from build123d import *

# Parameters (mm, degrees)
F0_R           = 12.5
F1_DEPTH       = 122.5
F2_R           = 12.5
F3_DEPTH       = 65
F4_DEPTH       = 25
F5_DEPTH       = 25
F6_R           = 5.5
F7_DEPTH       = 30
F9_D           = 5.5
F9_DEPTH       = 100
F9_CSINK_D     = 11
F9_CSINK_ANGLE = 90


with BuildPart() as f1:
    # F0 (on Top) → F1 (new body)
    with BuildSketch(Plane.XY):
        Circle(F0_R)
    extrude(amount=F1_DEPTH)

    # F2 (on Right) → F3 (join)
    with BuildSketch(Plane.YZ):
        Circle(F2_R)
    extrude(amount=F3_DEPTH)

    # F2 (on Right) → F4 (join)
    with BuildSketch(Plane.YZ):
        Circle(F2_R)
    extrude(amount=-F4_DEPTH)

    # F0 (on Top) → F5 (join)
    with BuildSketch(Plane.XY):
        Circle(F0_R)
    extrude(amount=-F5_DEPTH)

    # F6 (on face) → F7 (cut)
    with BuildSketch(Plane(origin=(-25, 0, 0), x_dir=(0, -1, 0), z_dir=(-1, 0, 0))):
        Circle(F6_R)
    extrude(amount=-F7_DEPTH, mode=Mode.SUBTRACT)

    # F9
    with Locations(Plane(origin=(5, 0, 0), x_dir=(0, -1, 0), z_dir=(-1, 0, 0))):
        with Locations((0, 0)):
            CounterSinkHole(F9_D / 2, F9_CSINK_D / 2, depth=F9_DEPTH, counter_sink_angle=F9_CSINK_ANGLE)


solid = f1.part
Model file for the job. Use its own axes, mm. A direction names the side the tool comes from. Give positions to 0.01 mm unless a question says otherwise; leave off trailing zeros. Loops run counter-clockwise (first coordinate to the right, second up) from the corner with the lowest first, then second, coordinate; pieces in that order, holes last.
Item 1: Drop flat-ended pins along their axis: P1, Ø3.5, axis at y = 0, z = 0, coming from the -X side (3 decimals); P2, Ø5, axis at x = 21.5, y = 9.5, coming from the +Z side; P3, Ø3, axis at y = 5, z = 43, coming from the -X side; P4, Ø2, axis at x = 13, y = -4.5, coming from the +Z side. Give the stop position or say it passes through.
Check values:
P1: passes through
P2: stops at z = 10.36
P3: stops at x = -12
P4: stops at z = 12
Item 2: Mould opens along Y. For faces 5 (the face through (0, 0, 122.5)), 6 (the face through (-10.21, 1.19, -5.37)), 7 (the face through (-15.103, -9.92, -7.606)) say: +Y half, -Y half, draft (parallel to the pull), parting line (faces both ways), or undercut.
Check values:
face 5: draft
face 6: undercut
face 7: parting line
Item 3: Slice it at D-D (z = 87). Write the cut outline in (x, y).
Check values:
outline: circle Ø25 at (0, 0)
Item 4: Drill centre lines: line 1 along Z through (x, y) = (-17.25, 0); line 2 along Z through (x, y) = (-11.5, 0); line 3 along X through (y, z) = (-0.5, 105). Where is each one in solid material? Low to high.
Check values:
line 1: z = -12.5 to -5.5, 5.5 to 12.5
line 2: z = -25 to -5.5, 5.5 to 122.5
line 3: x = -12.49 to 12.49
Item 5: Slice it at B-B (x = -18.5). Write the cut outline in (y, z).
Check values:
outline: circle Ø25 at (0, 0); hole circle Ø11 at (0, 0)
Item 6: Slice it at A-A (y = 0). Write the cut outline in (x, z), plus the area to 3 significant figures.
Check values:
outline: (-25, -12.5) - (-12.5, -12.5) - (-12.5, -25) - (12.5, -25) - (12.5, -12.5) - (65, -12.5) - (65, -2.75) - (7.75, -2.75) - (5, -5.5) - (-25, -5.5) - close; (-25, 5.5) - (5, 5.5) - (7.75, 2.75) - (65, 2.75) - (65, 12.5) - (12.5, 12.5) - (12.5, 122.5) - (-12.5, 122.5) - (-12.5, 12.5) - (-25, 12.5) - close
area: 4,640 mm2
Item 7: Slice it at C-C (y = -9.75). Write the cut outline in (x, z).
Check values:
outline: (-25, -7.82) - (-7.82, -7.82) - (-7.82, -25) - (7.82, -25) - (7.82, -7.82) - (65, -7.82) - (65, 7.82) - (7.82, 7.82) - (7.82, 122.5) - (-7.82, 122.5) - (-7.82, 7.82) - (-25, 7.82) - close
Item 8: Which spindle directions (+Z, -Z, +X, -X, +Y, -Y) get a long thin tool onto all of the face, cutting with end or side? Do faces 1 (the face through (7.62, -0.63, -2.81)), 2 (the face through (39.267, -12.488, 0.55)), 3 (the face through (11.923, 3.755, -15.103)), 4 (the face through (5.77, -11.09, 60.39)). Say none if no direction does.
Check values:
face 1: -X
face 2: +X
face 3: -Z
face 4: +Z
